Geometry: see drawing. Coordinates: mm, zero at the bounding-box minimum. Round coordinates to 2 decimals unless told otherwise and drop trailing zeros. Write each loop counter-clockwise with the first axis right and the second up, starting at its lowest first coordinate (ties: lowest second). Pieces come first, ordered by that corner, then holes. Notation, with made-up numbers: M -19.5,71.25 L -10.5,71.25 A37 ccw -10.5,107.25 Z; hole C -31,-16 d7. An arc over 180 degrees is marked long. Use a Markdown table: item, result.
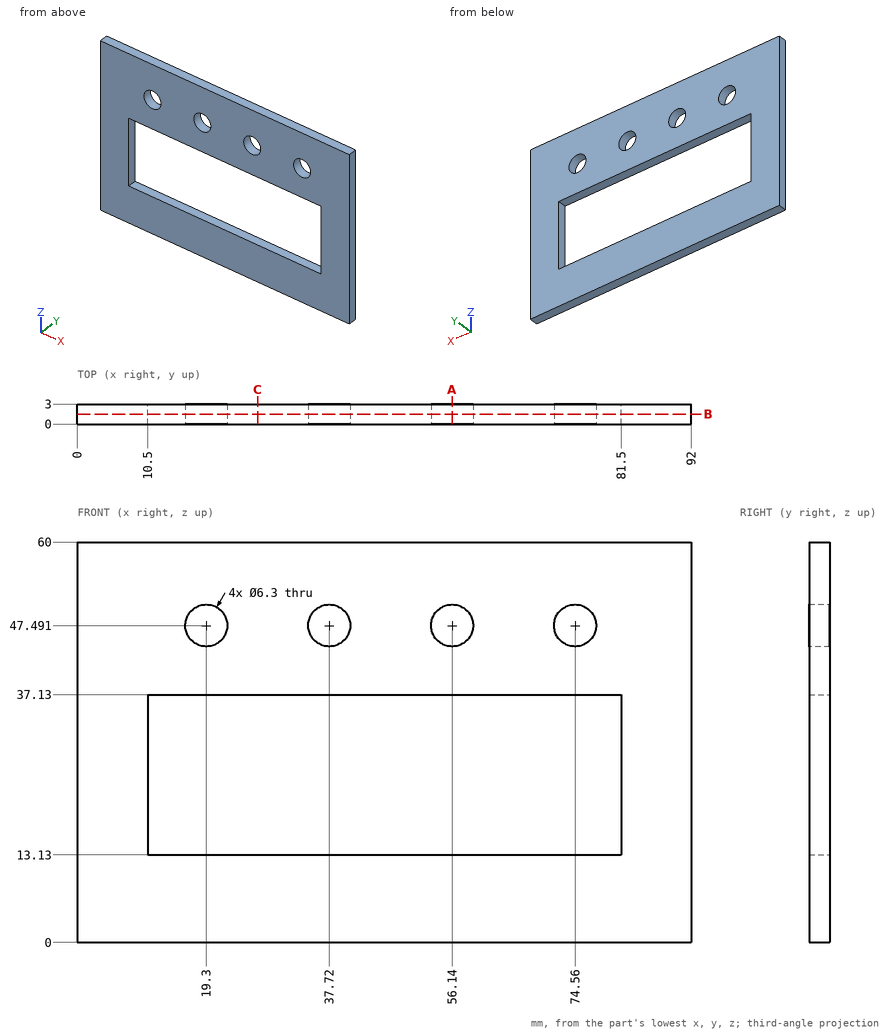
Q1. Line query: L1, parallel to Z at x = 19.5, y = 1.4; L2, parallel to X at y = 2.35, z = 26.5; L3, parallel to Z at x = 66, y = 2.55. Output: solid intervals per line, ascending.
Results are:
| item | result |
|---|---|
| L1 | 0 to 13.13, 37.13 to 44.35, 50.63 to 60 |
| L2 | 0 to 10.5, 81.5 to 92 |
| L3 | 0 to 13.13, 37.13 to 60 |
Q2. Section A-A on x = 56.14. Return loops of the section in (y, z), plus the area to 3 significant figures.
Results are:
| item | result |
|---|---|
| outline | M 0,0 L 3,0 L 3,13.13 L 0,13.13 Z; M 0,37.13 L 3,37.13 L 3,44.34 L 0,44.34 Z; M 0,50.64 L 3,50.64 L 3,60 L 0,60 Z |
| area | 89.1 mm^2 |
Q3. Section B-B on y = 1.5. Return loops of the section in (x, z).
Results are:
| item | result |
|---|---|
| outline | M 0,0 L 92,0 L 92,60 L 0,60 Z; hole M 10.5,13.13 L 81.5,13.13 L 81.5,37.13 L 10.5,37.13 Z; hole C 19.3,47.49 d6.3; hole C 37.72,47.49 d6.3; hole C 56.14,47.49 d6.3; hole C 74.56,47.49 d6.3 |
Q4. First-contact query: pin 1 Ø10 at (x, z) = (56.14, 47.49) entering from -Y. Flat tip, straight axial feed; report the tip coordinate or a pass-through.
Results are:
| item | result |
|---|---|
| pin 1 | y = 0 |
Q5. Section C-C on x = 27. Return loops of the section in (y, z), plus the area to 3 significant figures.
Results are:
| item | result |
|---|---|
| outline | M 0,0 L 3,0 L 3,13.13 L 0,13.13 Z; M 0,37.13 L 3,37.13 L 3,60 L 0,60 Z |
| area | 108 mm^2 |
